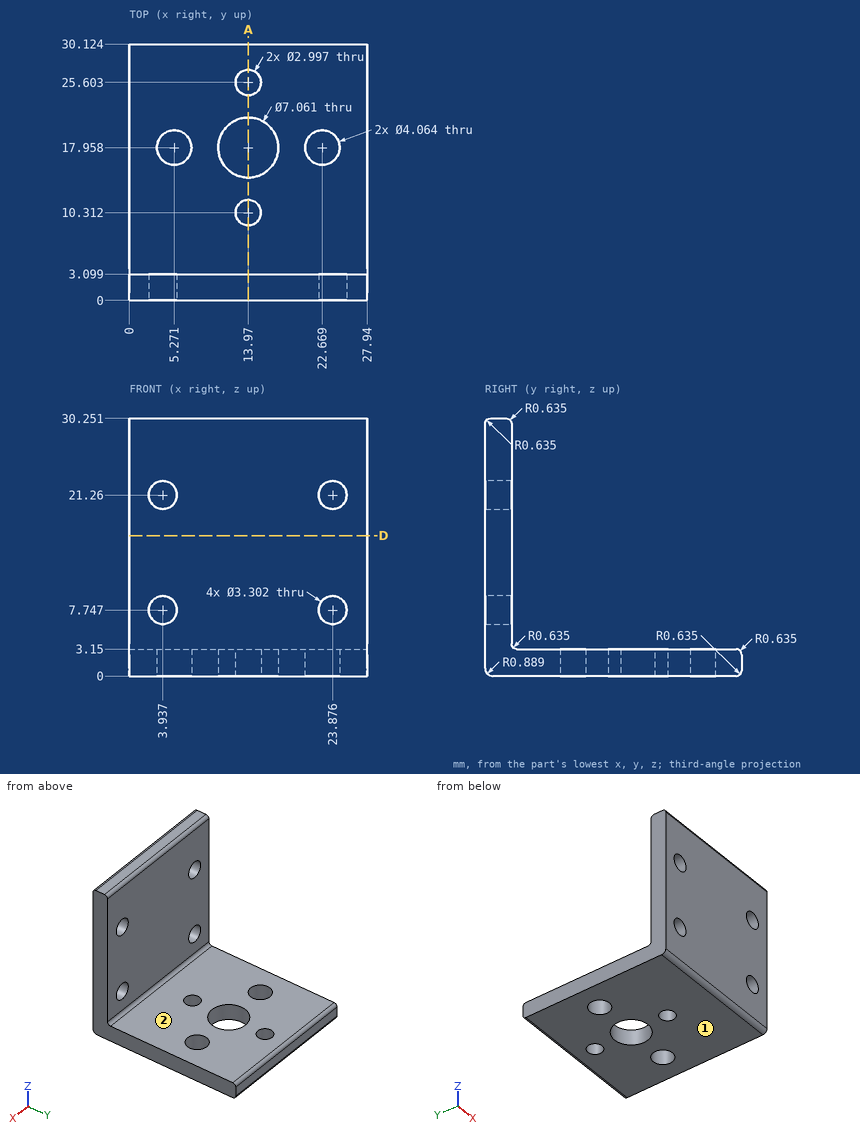
Input: dimensioned drawing with shaded views. Units: mm. Origin: part minimum x, y, z. A direction names the side the tool comes from. Coordinates: 2 decimals unless noted, no trailing zeros. Order: outer loops, then holes, each group sorted by start corner. A loop starts at its lowest first (then second) coordinate and runs counter-clockwise, first axis right, second up. Notation, with made-up numbers: (89.25, 9) -> (128.25, 9) arc R15 ccw to (128.25, 36) -> close; hole circle Ø6 at (-37.5, 55). An arc over 180 degrees is marked (long way). Answer in a Markdown table with one row per item.
Item 1: Ray query, L1, parallel to Z at x = 10.75, y = 28; L2, parallel to Y at x = 2, z = 26.5; L3, parallel to X at y = 20.5, z = 2. Return the intervals inside material, ascending.
Return value:
| item | result |
|---|---|
| L1 | z = 0 to 3.15 |
| L2 | y = 0 to 3.1 |
| L3 | x = 0 to 11.52, 16.42 to 27.94 |
Item 2: Section D-D on z = 16.5. Output: boundary loops of the cut face in (x, y).
Return value:
| item | result |
|---|---|
| outline | (0, 0) -> (27.94, 0) -> (27.94, 3.1) -> (0, 3.1) -> close |
Item 3: Access query for the marked faces 1 and 2. Directions: +Z, -Z, +X, -X, +Y, -Y. A direction counts if a zero-diameter tool reaches every point of the face in a straight line with its end or side. Return the directions, or none.
Return value:
| item | result |
|---|---|
| face 1 | -Z, +X, -X, +Y, -Y |
| face 2 | +Z, +X, -X, +Y |
Item 4: Contact query for flat-ended pins moving along their axis: P1, Ø5.5, axis at x = 23.88, z = 21.26, coming from the +Y side; P2, Ø3, axis at x = 16.5, y = 8.5, coming from the +Z side; P3, Ø8, axis at x = 25, y = 6, coming from the +Z side. Output: stop coordinate, or through.
Return value:
| item | result |
|---|---|
| P1 | stops at y = 3.1 |
| P2 | stops at z = 3.15 |
| P3 | stops at z = 30.25 |
Item 5: Section A-A on x = 13.97. State how many separate pieces and enclosed holes the cut face has, plus the area to 3 significant figures.
Return value:
| item | result |
|---|---|
| separate pieces | 4 |
| enclosed holes | 0 |
| area | 137 mm² |
